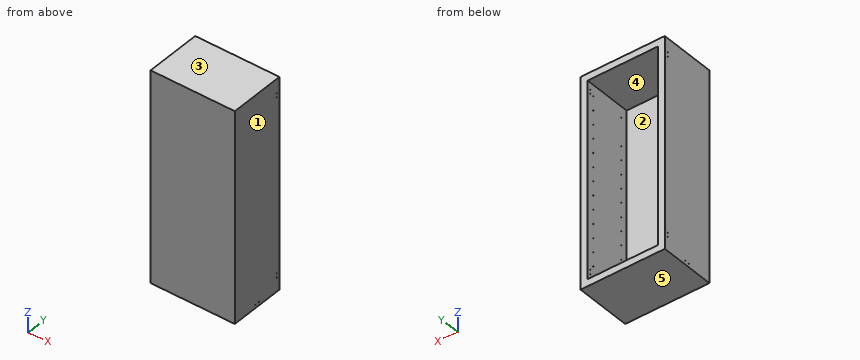
from build123d import *

# Parameters (mm, degrees)
SKETCH1_W           = 600
SKETCH1_H           = 1500
BOSS_EXTRUDE1_DEPTH = 400
SHELL1_T            = -50
SKETCH2_R           = 2.5
CUT_EXTRUDE1_DEPTH  = 1041.432602334
SKETCH13_R          = 2.5
CUT_EXTRUDE2_DEPTH  = 275
LPATTERN1_COUNT     = 13
LPATTERN1_PITCH     = 100
SKETCH14_R          = 2.5
CUT_EXTRUDE3_DEPTH  = 25


with BuildPart() as part:
    # Sketch1 → Boss-Extrude1 (new body)
    with BuildSketch(Plane(origin=(0, 0, 0), x_dir=(1, 0, 0), z_dir=(0, 1, 0))):
        Rectangle(SKETCH1_W, SKETCH1_H)
    extrude(amount=BOSS_EXTRUDE1_DEPTH)

    # Shell1
    shell1_openings = [part.faces().sort_by_distance(p)[0] for p in [
        (0, 400, 0),
    ]]
    offset(amount=SHELL1_T, openings=shell1_openings, kind=Kind.INTERSECTION)

    # Sketch2 → Cut-Extrude1 (cut, through all)
    with BuildSketch(Plane(origin=(300, 0, 0), x_dir=(0, 0, -1), z_dir=(1, 0, 0))):
        with Locations((-650, 375)):
            Circle(SKETCH2_R)
        with Locations((-620, 375)):
            Circle(SKETCH2_R)
        with Locations((650, 375)):
            Circle(SKETCH2_R)
        with Locations((620, 375)):
            Circle(SKETCH2_R)
    extrude(amount=-CUT_EXTRUDE1_DEPTH, mode=Mode.SUBTRACT)

    # Sketch13 → Cut-Extrude2 (cut, symmetric)
    with BuildSketch(Plane(origin=(0, 0, 0), x_dir=(0, 0, -1), z_dir=(1, 0, 0))):
        with Locations((-620, 350)):
            Circle(SKETCH13_R)
        with Locations((-620, 100)):
            Circle(SKETCH13_R)
    cut_extrude2 = extrude(amount=CUT_EXTRUDE2_DEPTH, both=True, mode=Mode.SUBTRACT)

    # LPattern1: Cut-Extrude2 ×13
    with Locations(*[(0, 0, -i * LPATTERN1_PITCH) for i in range(1, LPATTERN1_COUNT)]):
        add(cut_extrude2, mode=Mode.SUBTRACT)

    # Sketch14 → Cut-Extrude3 (cut)
    with BuildSketch(Plane(origin=(300, 0, 0), x_dir=(0, 0, -1), z_dir=(1, 0, 0))):
        with Locations((725, 215)):
            Circle(SKETCH14_R)
        with Locations((725, 185)):
            Circle(SKETCH14_R)
    cut_extrude3 = extrude(amount=-CUT_EXTRUDE3_DEPTH, mode=Mode.SUBTRACT)

    # Mirror1: Cut-Extrude3 across plane
    add(cut_extrude3.mirror(Plane(origin=(0, 0, 0), x_dir=(0, 0, 1), z_dir=(1, 0, 0))), mode=Mode.SUBTRACT)


solid = part.part
Can you work these out from the model? Positions are in its coordinate system, mm. Face numbers are marked on the shaded views. A direction names the side the tool comes from. Coordinates: 2 decimals unless noted, no trailing zeros. Write each loop counter-clockwise with the first axis right and the second up, starting at its lowest first coordinate (ties: lowest second). Pieces come first, ordered by that corner, then holes.
Q1. For P1, Ø12, axis at x = 125.5, z = 29.5, coming from the +Y side, with a flat end and sliding along its axis, tell me the tip position at first contact or that it passes through.
Results found:
P1: stops at y = 50
Q2. Imagine slicing it at B-B, the plane z = 349. List the corners of the cut face in (x, y) for me.
Results found:
outline: (-300, 0) - (300, 0) - (300, 400) - (250, 400) - (250, 50) - (-250, 50) - (-250, 400) - (-300, 400) - close
Q3. Imagine slicing it at A-A, the plane y = 83.5. List the corners of the cut face in (x, z) for me.
Results found:
outline: (-300, -750) - (300, -750) - (300, 750) - (-300, 750) - close; hole (-250, -700) - (250, -700) - (250, 700) - (-250, 700) - close
Q4. Imagine slicing it at C-C, the plane x = 67.5. List the corners of the cut face in (y, z) for me, plus the area to 3 significant figures.
Results found:
outline: (0, -750) - (400, -750) - (400, -700) - (50, -700) - (50, 700) - (400, 700) - (400, 750) - (0, 750) - close
area: 110,000 mm2
Q5. Please list where these lines run through material, in increasing order: L1, parallel to Y at x = -266, z = -380; L2, parallel to Y at x = -272, z = 620; L3, parallel to Z at x = 38, y = 307.
Results found:
L1: y = 0 to 97.5, 102.5 to 347.5, 352.5 to 400
L2: y = 0 to 97.5, 102.5 to 347.5, 352.5 to 372.5, 377.5 to 400
L3: z = -750 to -700, 700 to 750
Q6. Which directions (+Z, -Z, +X, -X, +Y, -Y) give clear straight access to the entire face, cutting with the end or side of a thin tool? Please do the marked faces 4 and 5.
Results found:
face 4: +Y
face 5: -Z, +X, -X, +Y, -Y
Q7. If we mould it in two halves opening along X, with no side actions, what happens to the marked faces 1, 2 and 3? For each: +X half, -X half, draft (parallel to the pull), parting line (faces both ways), or undercut.
Results found:
face 1: +X half
face 2: undercut
face 3: draft
